```python
from build123d import *
from build123d.topology import SkipClean

# Parameters (mm, degrees)
SKETCH1_W                   = 32.65
SKETCH1_H                   = 81.2
BOSS_EXTRUDE1_DEPTH         = 1
BOSS_EXTRUDE2_DEPTH         = 4
SKETCH3_W                   = 5.2
SKETCH3_H                   = 5.2
BOSS_EXTRUDE3_DEPTH         = 1
F_3DSKETCH1_R               = 2
CUT_EXTRUDE13_DEPTH         = 15
F_3DSKETCH2_R               = 2.6
CUT_EXTRUDE14_DEPTH         = 24
CUT_EXTRUDE20_START         = -6.9
SKETCH7_R                   = 2
CUT_EXTRUDE20_DEPTH         = 6.9
SKETCH8_W                   = 1
SKETCH8_H                   = 5
CUT_EXTRUDE21_DEPTH         = 88.661066044
SKETCH9_W                   = 5
SKETCH9_H                   = 1
CUT_EXTRUDE23_DEPTH         = 87.935967815
SKETCH11_W                  = 10
SKETCH11_H                  = 6
BOSS_EXTRUDE4_DEPTH         = 3
TAP_DRILL_FOR_M2X0_4_TAP1_D = 1.6
TAP_DRILL_FOR_M2X0_4_TAP2_D = 1.6
SKETCH37_R                  = 0.8
BOSS_EXTRUDE11_DEPTH        = 1
SKETCH40_W                  = 2.3
SKETCH40_H                  = 65
BOSS_EXTRUDE12_DEPTH        = 1
SKETCH41_W                  = 26.05
SKETCH41_H                  = 7.4
BOSS_EXTRUDE13_DEPTH        = 1
M3_CLEARANCE_HOLE1_D        = 3.4
M3_CLEARANCE_HOLE2_D        = 3.4


with BuildPart() as part:
    # Sketch1 → Boss-Extrude1 (new body)
    with BuildSketch(Plane.XY):
        with Locations((16.325, 40.6)):
            Rectangle(SKETCH1_W, SKETCH1_H)
    extrude(amount=BOSS_EXTRUDE1_DEPTH)

    # Sketch2 → Boss-Extrude2 (add)
    with BuildSketch(Plane.XY.offset(1)):
        Polygon((0, 0), (0, 81.2), (32.65, 81.2), (32.65, 0), (31.65, 0), (31.65, 80.2), (1, 80.2), (1, 0), align=None)
    extrude(amount=BOSS_EXTRUDE2_DEPTH)

    # Sketch3 → Boss-Extrude3 (add)
    with BuildSketch(Plane.XY.offset(1)):
        with Locations((3.6, 77.6)):
            Rectangle(SKETCH3_W, SKETCH3_H)
        with Locations((3.6, 17.8)):
            Rectangle(SKETCH3_W, SKETCH3_H)
        with Locations((29.05, 17.8)):
            Rectangle(SKETCH3_W, SKETCH3_H)
        with Locations((29.05, 77.6)):
            Rectangle(SKETCH3_W, SKETCH3_H)
    extrude(amount=BOSS_EXTRUDE3_DEPTH)

    # 3DSketch1 → Cut-Extrude13 (cut)
    with BuildSketch(Plane(origin=(11.325, 80.2, 4), x_dir=(1, 0, 0), z_dir=(0, -1, 0))):
        Circle(F_3DSKETCH1_R)
        with Locations((10, 0)):
            Circle(F_3DSKETCH1_R)
    extrude(amount=-CUT_EXTRUDE13_DEPTH, mode=Mode.SUBTRACT)

    # 3DSketch2 → Cut-Extrude14 (cut)
    with BuildSketch(Plane(origin=(9.675, 61.1, 1), x_dir=(0.4145072564800623, -0.910046006708107, 0), z_dir=(0, 0, 1))):
        with Locations(Location((0, 0, 0), (0, 0, 245.511710088))):
            Circle(F_3DSKETCH2_R)
        with Locations(Location((5.512946511, 12.103611889, 0), (0, 0, 245.511710088))):
            Circle(F_3DSKETCH2_R)
        with Locations(Location((6.82534505, -3.108804424, 0), (0, 0, 245.511710088))):
            Circle(F_3DSKETCH2_R)
        with Locations(Location((12.338291561, 8.994807466, 0), (0, 0, 245.511710088))):
            Circle(F_3DSKETCH2_R)
        with Locations(Location((20.021012148, -9.119159643, 0), (0, 0, 245.511710088))):
            Circle(F_3DSKETCH2_R)
        with Locations(Location((25.533958659, 2.984452247, 0), (0, 0, 245.511710088))):
            Circle(F_3DSKETCH2_R)
        with Locations(Location((26.573343396, -12.103611889, 0), (0, 0, 245.511710088))):
            Circle(F_3DSKETCH2_R)
        with Locations(Location((32.086289907, 0, 0), (0, 0, 245.511710088))):
            Circle(F_3DSKETCH2_R)
    extrude(amount=-CUT_EXTRUDE14_DEPTH, mode=Mode.SUBTRACT)

    # Sketch7 → Cut-Extrude20 (cut)
    with BuildSketch(Plane(origin=(0, 81.2, 0), x_dir=(1, 0, 0), z_dir=(0, 1, 0)).offset(CUT_EXTRUDE20_START)):
        with BuildLine():
            ThreePointArc((13.057050808, -5), (13.256851653, -4.51763809), (13.325, -4))
            ThreePointArc((13.325, -4), (10.80736191, -2.068148347), (9.592949192, -5))
            Line((9.592949192, -5), (13.057050808, -5))
        make_face()
        with BuildLine():
            Line((13.057050808, -5), (9.592949192, -5))
            ThreePointArc((9.592949192, -5), (11.325, -6), (13.057050808, -5))
        make_face()
        with BuildLine():
            ThreePointArc((9.592949192, -5), (11.325, -2), (13.057050808, -5))
            Line((13.057050808, -5), (9.592949192, -5))
        make_face()
        with Locations((21.308255446, -4.002965824)):
            Circle(SKETCH7_R)
    extrude(amount=CUT_EXTRUDE20_DEPTH, mode=Mode.SUBTRACT)

    # Sketch8 → Cut-Extrude21 (cut, through all)
    with BuildSketch(Plane.XZ):
        Polygon((1, 5), (0, 5), (0, 0), (1, 0), (1, 1), align=None)
        with Locations((32.15, 2.5)):
            Rectangle(SKETCH8_W, SKETCH8_H)
    extrude(amount=-CUT_EXTRUDE21_DEPTH, mode=Mode.SUBTRACT)

    # Sketch9 → Cut-Extrude23 (cut, through all)
    with BuildSketch(Plane(origin=(31.65, 0, 0), x_dir=(0, 0, -1), z_dir=(1, 0, 0))):
        with Locations((-2.5, 80.7)):
            Rectangle(SKETCH9_W, SKETCH9_H)
    extrude(amount=-CUT_EXTRUDE23_DEPTH, mode=Mode.SUBTRACT)

    # Sketch11 → Boss-Extrude4 (add)
    with BuildSketch(Plane(origin=(0, 0, 0), x_dir=(-1, 0, 0), z_dir=(0, 0, -1))):
        with Locations((-26.65, 18)):
            Rectangle(SKETCH11_W, SKETCH11_H)
        with Locations((-26.65, 70.2)):
            Rectangle(SKETCH11_W, SKETCH11_H)
        with Locations((-6, 70.2)):
            Rectangle(SKETCH11_W, SKETCH11_H)
        with Locations((-6, 18)):
            Rectangle(SKETCH11_W, SKETCH11_H)
    extrude(amount=BOSS_EXTRUDE4_DEPTH)

    # Tap Drill for M2x0.4 Tap1 (through all)
    with Locations(Plane(origin=(26.675, 70.1, 2), x_dir=(1, 0, 0), z_dir=(0, 0, 1))):
        with Locations((0, 0)):
            Hole(TAP_DRILL_FOR_M2X0_4_TAP1_D / 2)

    # Tap Drill for M2x0.4 Tap2 (through all)
    with Locations(Plane(origin=(5.975, 70.1, 2), x_dir=(1, 0, 0), z_dir=(0, 0, 1))):
        with Locations((0, 0), (0, -52.15), (20.702261821, -52.15)):
            Hole(TAP_DRILL_FOR_M2X0_4_TAP2_D / 2)

    # Sketch37 → Boss-Extrude11 (add)
    with SkipClean():  # the faces are left unmerged after this step: merging them gives an invalid solid
        with BuildSketch(Plane.XY.offset(1)):
            with BuildLine():
                Line((26.85, 64.95), (26.85, 27.95))
                Line((26.85, 27.95), (19.475, 27.95))
                Line((19.475, 27.95), (19.475, 15.2))
                Line((19.475, 15.2), (26.45, 15.2))
                Line((26.45, 15.2), (26.45, 17.18295889))
                ThreePointArc((26.45, 17.18295889), (25.877261821, 17.95), (26.45, 18.71704111))
                Line((26.45, 18.71704111), (26.45, 20.4))
                Line((26.45, 20.4), (31.65, 20.4))
                Line((31.65, 20.4), (31.65, 75))
                Line((31.65, 75), (26.45, 75))
                Line((26.45, 75), (26.45, 80.2))
                Line((26.45, 80.2), (6.2, 80.2))
                Line((6.2, 80.2), (6.2, 75))
                Line((6.2, 75), (1, 75))
                Line((1, 75), (1, 20.4))
                Line((1, 20.4), (6.2, 20.4))
                Line((6.2, 20.4), (6.2, 18.717707627))
                ThreePointArc((6.2, 18.717707627), (6.775, 17.95), (6.2, 17.182292373))
                Line((6.2, 17.182292373), (6.2, 15.2))
                Line((6.2, 15.2), (13.225, 15.2))
                Line((13.225, 15.2), (13.225, 27.95))
                Line((13.225, 27.95), (5.85, 27.95))
                Line((5.85, 27.95), (5.85, 64.95))
                Line((5.85, 64.95), (26.85, 64.95))
            make_face()
            with Locations((5.975, 70.1)):
                Circle(SKETCH37_R, mode=Mode.SUBTRACT)
            with Locations((26.675, 70.1)):
                Circle(SKETCH37_R, mode=Mode.SUBTRACT)
        extrude(amount=BOSS_EXTRUDE11_DEPTH)
    add(part.part.scale(1), mode=Mode.REPLACE)  # the faces are merged on a copy

    # Sketch40 → Boss-Extrude12 (add)
    with BuildSketch(Plane.XY.offset(2)):
        with Locations((30.5, 47.7)):
            Rectangle(SKETCH40_W, SKETCH40_H)
        with Locations((2.15, 47.7)):
            Rectangle(SKETCH40_W, SKETCH40_H)
    extrude(amount=BOSS_EXTRUDE12_DEPTH)

    # Sketch41 → Boss-Extrude13 (add)
    with BuildSketch(Plane.XY.offset(2)):
        with Locations((16.325, 76.5)):
            Rectangle(SKETCH41_W, SKETCH41_H)
    extrude(amount=BOSS_EXTRUDE13_DEPTH)

    # M3 Clearance Hole1 (through all)
    with Locations(Plane(origin=(4.5, 76.7, 3), x_dir=(1, 0, 0), z_dir=(0, 0, 1))):
        with Locations((0, 0), (23.65, 0)):
            Hole(M3_CLEARANCE_HOLE1_D / 2)

    # M3 Clearance Hole2 (through all)
    with Locations(Plane(origin=(6.925, 22.85, 2), x_dir=(1, 0, 0), z_dir=(0, 0, 1))):
        with Locations((0, 0), (18.8, 0)):
            Hole(M3_CLEARANCE_HOLE2_D / 2)


solid = part.part
```
The listing builds one solid part. Answer for the finished solid, in the listing's coordinates (mm). A direction names the side the tool comes from. Coordinates: 2 decimals unless noted, no trailing zeros. Write each loop counter-clockwise with the first axis right and the second up, starting at its lowest first coordinate (ties: lowest second). Pieces come first, ordered by that corner, then holes. Notation, with made-up numbers: (11.5, -23.75) - (51.5, -23.75) arc R12 ccw to (51.5, -19.75) - close; hole circle Ø8 at (-3, 15.25). An arc over 180 degrees is marked (long way). Return JSON: item names as keys, results as strings. Group by question number.
Q1. For a pull along X with two mould halves and no side action, classify faces 4 (the flat face through (5.7, 15.2, 1.8)), 5 (the flat face through (21.65, 18, -1)), 6 (the flat face through (31.65, 48, 1)) as +X half, -X half, draft (parallel to the pull), parting line (faces both ways), or undercut.
Q2. Which of the six approach directions +Z, -Z, +X, -X, +Y, -Y give full straight-line access (tool end or side, diameter ignored) to faces 1 (the flat face through (28, 44, 2)), 2 (the flat face through (27, 15, -1)), 3 (the flat face through (21.65, 70, -1))?
Q3. Flat-ended cylindrical pins translate along their axes: pin 1 Ø1.5 at (x, z) = (25, -1.5) entering from -Y; pin 2 Ø1.6 at (x, z) = (28.5, 2) entering from -Y; pin 3 Ø1.8 at (x, y) = (26.675, 70.1) entering from +Z. Find the tip coordinate at first contact, or state that the pin passes through.
Q4. Find the intervals of material crossed by line 1 along X through (y, z) = (17.95, -0.8) (3 decimals); line 2 along X through (y, z) = (39.1, 0.25) (3 decimals); line 3 along X through (y, z) = (70.1, 1.7) (3 decimals), in increasing order. Write a range as [from, to].
Q5. The part is cut by section D-D on x = 23. State how many separate pieces and enclosed holes the cut face has, and give its area (3 significant figures).
Q6. The part is cut by section C-C on y = 61.1. Write down the section's boundary in (x, z) (3 decimals), and give its area (3 significant figures).
Q7. The part is cut by section A-A on y = 70.1. Write down the section's boundary in (x, z) (3 decimals), and give its area (3 significant figures).
Q8. The part is cut by section B-B on x = 15. Write down the section's boundary in (y, z), and give its area (3 significant figures).
Evaluation:
{
 "1": {"face 4": "draft", "face 5": "undercut", "face 6": "+X half"},
 "2": {"face 1": "+Z, -Y", "face 2": "-Z, +X, -X, -Y", "face 3": "-Z, +Y, -Y"},
 "3": {"pin 1": "stops at y = 15", "pin 2": "stops at y = 15.2", "pin 3": "stops at z = 2"},
 "4": {"line 1": "x = [1, 5.175], [6.775, 11], [21.65, 25.877], [27.477, 31.65]", "line 2": "x = [1, 7.075], [12.275, 20.375], [25.575, 31.65]", "line 3": "x = [1, 5.175], [6.775, 25.875], [27.475, 31.65]"},
 "5": {"separate pieces": "5", "enclosed holes": "0", "area": "131 mm2"},
 "6": {"outline": "(1, 0) - (7.075, 0) - (7.075, 1) - (5.85, 1) - (5.85, 2) - (3.3, 2) - (3.3, 3) - (1, 3) - close; (12.275, 0) - (20.375, 0) - (20.375, 1) - (12.275, 1) - close; (25.575, 0) - (31.65, 0) - (31.65, 3) - (29.35, 3) - (29.35, 2) - (26.85, 2) - (26.85, 1) - (25.575, 1) - close", "area": "34.5 mm2"},
 "7": {"outline": "(1, -3) - (5.175, -3) - (5.175, 2) - (3.3, 2) - (3.3, 3) - (1, 3) - close; (6.775, -3) - (11, -3) - (11, 0) - (21.65, 0) - (21.65, -3) - (25.875, -3) - (25.875, 2) - (6.775, 2) - close; (27.475, -3) - (31.65, -3) - (31.65, 3) - (29.35, 3) - (29.35, 2) - (27.475, 2) - close", "area": "110 mm2"},
 "8": {"outline": "(0, 0) - (80.2, 0) - (80.2, 3) - (72.8, 3) - (72.8, 2) - (64.95, 2) - (64.95, 1) - (0, 1) - close", "area": "103 mm2"}
}
